Here's how the part is built. I have some questions about the finished solid (model axes, mm). A direction names the side the tool comes from. Round coordinates to 2 decimals unless told otherwise and drop trailing zeros. Write each loop counter-clockwise with the first axis right and the second up, starting at its lowest first coordinate (ties: lowest second). Pieces come first, ordered by that corner, then holes. Notation, with made-up numbers: M 59,-34.5 L 116,-34.5 A31 cw 116,-3.5 Z; hole C -36.75,-7.5 d2. An arc over 180 degrees is marked long. Write item = value, one per line. Start each with the question number.
(1) I want a section at A-A (x = -42). List the corners of the cut face in (y, z) for me, and give its area (3 significant figures).
(2) I want a section at C-C (y = 33.5). List the corners of the cut face in (x, z) for me, and give its area (3 significant figures).
(3) If we mould it in two halves opening along Z, with no side actions, what happens to faces 1 (the flat face through (-21.5, 20, 1)), 2 (the flat face through (-39, 3, 22)), 3 (the flat face through (-23, 2, 50)), 4 (the flat face through (45, 3, -23))? For each: released by +Z, released by -Z, zero draft, split by the parting line, or undercut.
(4) I want a section at B-B (z = 4.5). List the corners of the cut face in (x, y) for me, and give its area (3 significant figures).
(5) I need wall thicknesses on line 1 along X through (y, z) = (9, 29); line 2 along Z through (x, y) = (-28.5, 9.5); line 3 along Y through (x, z) = (42.5, 42.5). Which ranges of each line are inside material? Lowest first, please.
(6) Will these pins go through, and if not, where does the flat tip stop? pin 1 Ø5.5 at (y, z) = (2, 46) entering from -X; pin 2 Ø3 at (x, z) = (28, -18.5) entering from +Y; pin 3 Ø5 at (y, z) = (18, -9.5) entering from -X.
(7) On a 3-axis mill with a long thin cutter (end or side, diameter ignored), from which of +Z, -Z, +X, -X, +Y, -Y can I reach the whole of each face in a straight line? I mean faces 5 (the flat face through (28, 10, 40)), 6 (the cylindrical face through (-41.9, 2.5, 35.5)), 7 (the flat face through (-21.5, 16, -17)). Say none if no direction works.
(8) I want a section at D-D (z = 16). Give the number of separate pieces and of enclosed holes in the cut face, and give its area (3 significant figures).
```python
from build123d import *

# Parameters (mm, degrees)
CROQUIS2_W              = 100
CROQUIS2_H              = 100
SALIENTE_EXTRUIR1_DEPTH = 5
REDONDEO1_R             = 10
CORTAR_EXTRUIR1_DEPTH   = 5
CROQUIS4_W              = 10
CROQUIS4_H              = 80
SALIENTE_EXTRUIR2_DEPTH = 40
CORTAR_EXTRUIR2_DEPTH   = 84
SALIENTE_EXTRUIR4_START = 2.5
SALIENTE_EXTRUIR4_DEPTH = 2.5
SALIENTE_EXTRUIR5_DEPTH = 2.5


with BuildPart() as part:
    # Croquis2 → Saliente-Extruir1 (new body)
    with BuildSketch(Plane(origin=(0, 0, 0), x_dir=(1, 0, 0), z_dir=(0, 1, 0))):
        Rectangle(CROQUIS2_W, CROQUIS2_H)
    extrude(amount=SALIENTE_EXTRUIR1_DEPTH)

    # Redondeo1
    redondeo1_edges = [part.edges().sort_by_distance(p)[0] for p in [
        (-50, 2.5, -50),
        (50, 2.5, -50),
        (50, 2.5, 50),
        (-50, 2.5, 50),
    ]]
    fillet(redondeo1_edges, radius=REDONDEO1_R)

    # Croquis3 → Cortar-Extruir1 (cut)
    with BuildSketch(Plane(origin=(0, 5, 0), x_dir=(1, 0, 0), z_dir=(0, 1, 0))):
        with BuildLine():
            Line((-5, -50), (5, -50))
            Line((5, -50), (5, -40))
            ThreePointArc((5, -40), (0, -35), (-5, -40))
            Line((-5, -40), (-5, -50))
        make_face()
        with BuildLine():
            Line((-39, 32.5), (-39, 12.5))
            ThreePointArc((-39, 12.5), (-42, 9.5), (-45, 12.5))
            Line((-45, 12.5), (-45, 32.5))
            ThreePointArc((-45, 32.5), (-42, 35.5), (-39, 32.5))
        make_face()
        with BuildLine():
            Line((45, 32.5), (45, 12.5))
            ThreePointArc((45, 12.5), (42, 9.5), (39, 12.5))
            Line((39, 12.5), (39, 32.5))
            ThreePointArc((39, 32.5), (42, 35.5), (45, 32.5))
        make_face()
        with BuildLine():
            Line((-39, -12.5), (-39, -32.5))
            ThreePointArc((-39, -32.5), (-42, -35.5), (-45, -32.5))
            Line((-45, -32.5), (-45, -12.5))
            ThreePointArc((-45, -12.5), (-42, -9.5), (-39, -12.5))
        make_face()
        with BuildLine():
            Line((45, -12.5), (45, -32.5))
            ThreePointArc((45, -32.5), (42, -35.5), (39, -32.5))
            Line((39, -32.5), (39, -12.5))
            ThreePointArc((39, -12.5), (42, -9.5), (45, -12.5))
        make_face()
        Polygon((0, 20.207259422), (-17.5, 10.103629711), (-17.5, -10.103629711), (0, -20.207259422), (17.5, -10.103629711), (17.5, 10.103629711), align=None)
    extrude(amount=-CORTAR_EXTRUIR1_DEPTH, mode=Mode.SUBTRACT)

    # Croquis4 → Saliente-Extruir2 (add)
    with BuildSketch(Plane(origin=(0, 5, 0), x_dir=(1, 0, 0), z_dir=(0, 1, 0))):
        with Locations((-29, 0)):
            Rectangle(CROQUIS4_W, CROQUIS4_H)
        with Locations((29, 0)):
            Rectangle(CROQUIS4_W, CROQUIS4_H)
    extrude(amount=SALIENTE_EXTRUIR2_DEPTH)

    # Croquis5 → Cortar-Extruir2 (cut)
    with BuildSketch(Plane(origin=(34, 0, 0), x_dir=(0, 0, -1), z_dir=(1, 0, 0))):
        with BuildLine():
            Line((-40, 15), (-35, 15))
            ThreePointArc((-35, 15), (1.310440846, 21.744044834), (30, 45))
            Line((30, 45), (-40, 45))
            Line((-40, 45), (-40, 15))
        make_face()
    extrude(amount=-CORTAR_EXTRUIR2_DEPTH, mode=Mode.SUBTRACT)

    # Croquis8 → Saliente-Extruir4 (add)
    with BuildSketch(Plane(origin=(-24, 0, 0), x_dir=(0, 0, -1), z_dir=(1, 0, 0)).offset(SALIENTE_EXTRUIR4_START)):
        with BuildLine():
            Line((-40, 12.973487285), (-40, 15))
            Line((-40, 15), (-35, 15))
            ThreePointArc((-35, 15), (1.310440846, 21.744044834), (30, 45))
            Line((30, 45), (33.091320679, 45))
            ThreePointArc((33.091320679, 45), (0.984523571, 18.856312683), (-40, 12.973487285))
        make_face()
    saliente_extruir4 = extrude(amount=-SALIENTE_EXTRUIR4_DEPTH)

    # Croquis9 → Saliente-Extruir5 (add)
    with BuildSketch(Plane(origin=(-24, 0, 0), x_dir=(0, 0, -1), z_dir=(1, 0, 0))):
        with BuildLine():
            Line((-40, 10.453567004), (-40, 5))
            Line((-40, 5), (40, 5))
            Line((40, 5), (40, 45))
            Line((40, 45), (36.132755539, 45))
            ThreePointArc((36.132755539, 45), (2.938227405, 16.990296255), (-40, 10.453567004))
        make_face()
    saliente_extruir5 = extrude(amount=SALIENTE_EXTRUIR5_DEPTH)

    # Simetría1: Saliente-Extruir4, Saliente-Extruir5 across plane
    add(saliente_extruir4.mirror(Plane(origin=(0, 0, 0), x_dir=(0, 0, 1), z_dir=(1, 0, 0))))
    add(saliente_extruir5.mirror(Plane(origin=(0, 0, 0), x_dir=(0, 0, 1), z_dir=(1, 0, 0))))


solid = part.part
```
Returned:
q1.outline = M 0,-49.8 L 5,-49.8 L 5,-35.5 L 0,-35.5 Z; M 0,-9.5 L 5,-9.5 L 5,9.5 L 0,9.5 Z; M 0,35.5 L 5,35.5 L 5,49.8 L 0,49.8 Z
q1.area = 238 mm²
q2.outline = M -34,-40 L -21.5,-40 L -21.5,-26.68 L -24,-26.68 L -24,-23.1 L -21.5,-23.1 L -21.5,-19.39 L -34,-19.39 Z; M 21.5,-40 L 34,-40 L 34,-19.39 L 21.5,-19.39 L 21.5,-23.1 L 24,-23.1 L 24,-26.68 L 21.5,-26.68 Z
q2.area = 497 mm²
q3.face_1 = zero draft
q3.face_2 = undercut
q3.face_3 = released by +Z
q3.face_4 = undercut
q4.outline = M -50,0 L -17.5,0 L -17.5,5 L -21.5,5 L -21.5,14.05 L -24,14.05 L -24,16.7 L -21.5,16.7 L -21.5,19.35 L -34,19.35 L -34,5 L -50,5 Z; M 17.5,0 L 50,0 L 50,5 L 34,5 L 34,19.35 L 21.5,19.35 L 21.5,16.7 L 24,16.7 L 24,14.05 L 21.5,14.05 L 21.5,5 L 17.5,5 Z
q4.area = 671 mm²
q5.line_1 = -34 to -21.5, 21.5 to 34
q5.line_2 = -40 to 40
q5.line_3 = 0 to 5
q6.pin_1 = -49.46
q6.pin_2 = 34.05
q6.pin_3 = -34
q7.face_5 = +Z, +X, -X, +Y
q7.face_6 = +Y, -Y
q7.face_7 = +Z, -Z, +Y
q8.separate_pieces = 4
q8.enclosed_holes = 0
q8.area = 634 mm²
